Read the model definition and answer for the solid it produces. Units are mm, in the model's axes. A direction names the side the tool comes from. Round coordinates to 2 decimals unless told otherwise and drop trailing zeros. Loops run counter-clockwise (first coordinate to the right, second up) from the corner with the lowest first, then second, coordinate; pieces in that order, holes last. Notation, with made-up numbers: M 13,3.5 L 43,3.5 A25 ccw 43,25.5 Z; hole C -25.5,0 d5. An arc over 180 degrees is marked long. Write each question's results on one line, items separated by ' | '.
from build123d import *

# Parameters (mm, degrees)
F1_DEPTH = 30
F2_SIZE  = 1
F3_R     = 2
F4_W     = 24.5
F4_H     = 2.5
F6_W     = 24.5389966294
F6_H     = 2.5
F6_W_2   = 24.6412428096
F6_W_3   = 24.4367551059
F6_W_4   = 24.5
F6_H_2   = 2.25


with BuildPart() as f1:
    # F0 (on Front) → F1 (new body)
    with BuildSketch(Plane.XZ):
        Polygon((-6, 0), (0, 0), (0, 10.7777772923), (17.2222208352, 10.7777772923), (17.2222208352, 15.7777772923), (4.666664066, 15.7777772923), (-18, 15.7777772923), (-18, 6.7777772923), (-12, 6.7777772923), (-12, 10.7777772923), (-6, 10.7777772923), align=None)
    extrude(amount=F1_DEPTH)

    # F2
    f2_edges = [f1.edges().sort_by_distance(p)[0] for p in [
        (-0.38889, -30, 15.777777),
        (17.222221, -15, 15.777777),
        (-0.38889, 0, 15.777777),
        (-18, -15, 15.777777),
        (-12, -15, 6.777777),
        (-6, -15, 0),
    ]]
    chamfer(f2_edges, length=F2_SIZE)

    # F3
    f3_edges = [f1.edges().sort_by_distance(p)[0] for p in [
        (0, -15, 10.777777),
    ]]
    fillet(f3_edges, radius=F3_R)

    # F4 (on face) → F7 section 0
    with BuildSketch(Plane.XY.offset(15.7777772923)):
        with Locations((0.8522442952, -25.1817190625)):
            Rectangle(F4_W, F4_H)
    # F6 (on offset) → F7 section 1
    with BuildSketch(Plane.XY.offset(12.2777772923)):
        with Locations((1.4323252253, -25.75)):
            Rectangle(F6_W, F6_H)
    loft(mode=Mode.SUBTRACT)

    # F4 (on face) → F8 section 0
    with BuildSketch(Plane.XY.offset(15.7777772923)):
        with Locations((0.8801504448, -18.1817190625)):
            Rectangle(F4_W, F4_H)
    # F6 (on offset) → F8 section 1
    with BuildSketch(Plane.XY.offset(12.2777772923)):
        with Locations((1.3812021352, -18.75)):
            Rectangle(F6_W_2, F6_H)
    loft(mode=Mode.SUBTRACT)

    # F4 (on face) → F9 section 0
    with BuildSketch(Plane.XY.offset(15.7777772923)):
        with Locations((1.0807377696, -11.1817190625)):
            Rectangle(F4_W, F4_H)
    # F6 (on offset) → F9 section 1
    with BuildSketch(Plane.XY.offset(12.2777772923)):
        with Locations((1.1767121032, -11.75)):
            Rectangle(F6_W_3, F6_H)
    loft(mode=Mode.SUBTRACT)

    # F4 (on face) → F10 section 0
    with BuildSketch(Plane.XY.offset(15.7777772923)):
        with Locations((0.9722208352, -4.1817190625)):
            Rectangle(F4_W, F4_H)
    # F6 (on offset) → F10 section 1
    with BuildSketch(Plane.XY.offset(12.2777772923)):
        with Locations((0.9722208352, -4.625)):
            Rectangle(F6_W_4, F6_H_2)
    loft(mode=Mode.SUBTRACT)


solid = f1.part
Item 1: The part is cut by section B-B (z = 10). Determine the outline of the cut face in (x, y), plus the area to 3 significant figures.
Outcome:
outline: M -18,-30 L -12,-30 L -12,0 L -18,0 Z; M -6,-30 L 0.42,-30 L 0.42,0 L -6,0 Z | area: 373 mm2
Item 2: The mould has two halves that part along X. Classify faces 6 (the face through (-5, -30, 9)), 7 (the face through (-12.493, -14.79, 7.285)), 8 (the face through (-5.5, -14.8, 0.5)): pulls with the +X half, pulls with the -X half, needs draft (parallel to the pull), parting line crosses it, or undercut.
Outcome:
face 6: needs draft | face 7: undercut | face 8: pulls with the -X half
Item 3: Straight lines are drawn through the part: line 1 (X direction, y = -23.5, z = 8.5); line 2 (Y direction, x = -5, z = 12.75); line 3 (Z direction, x = 10, y = -15.75). For each, find the intervals that lie inside material, in ascending order.
Outcome:
line 1: x = -18 to -12, -6 to 0 | line 2: y = -30 to -26.92, -24.42 to -19.92, -17.42 to -12.92, -10.42 to -5.71, -3.42 to 0 | line 3: z = 10.78 to 15.78
Item 4: The part is cut by section C-C (x = -15). Determine the outline of the cut face in (y, z), plus the area to 3 significant figures.
Outcome:
outline: M -30,6.78 L 0,6.78 L 0,14.78 L -1,15.78 L -29,15.78 L -30,14.78 Z | area: 269 mm2
Item 5: The part is cut by section D-D (z = 1.5). Determine the outline of the cut face in (x, y).
Outcome:
outline: M -6,-30 L 0,-30 L 0,0 L -6,0 Z
Item 6: The part is cut by section A-A (y = -9). Determine the outline of the cut face in (x, z).
Outcome:
outline: M -18,6.78 L -13,6.78 L -12,7.78 L -12,10.78 L -6,10.78 L -6,1 L -5,0 L 0,0 L 0,8.78 A2 cw 2,10.78 L 17.22,10.78 L 17.22,14.78 L 16.22,15.78 L -17,15.78 L -18,14.78 Z
Item 7: For faces 1 (the face through (0, -15, 4)), 2 (the face through (-12, -15, 9)), 3 (the face through (-16, -15, 6.778)), 4 (the face through (1, -19, 12.278)), 5 (the face through (1.14, -3.22, 14)), determine the directions among +Z, -Z, +X, -X, +Y, -Y from which every point of the face is accessible in a straight line to the end or side of a thin tool.
Outcome:
face 1: -Z, +X, +Y, -Y | face 2: -Z, +Y, -Y | face 3: -Z, -X, +Y, -Y | face 4: none | face 5: +Z
Item 8: Flat-ended cylindrical pins translate along their axes: pin 1 (2.5 mm diameter, centred on x = -16.5, y = -13, fed in from -Z); pin 2 (2.5 mm diameter, centred on y = -18, z = 6, fed in from +X); pin 3 (1.5 mm diameter, centred on y = -10, z = 8.5, fed in from +X). Find the tip coordinate at first contact, or state that the pin passes through.
Outcome:
pin 1: stops at z = 6.78 | pin 2: stops at x = 0 | pin 3: stops at x = 0.06
